Verification items for the finished model (mm, model axes). A direction names the side the tool comes from. Round coordinates to 2 decimals unless told otherwise and drop trailing zeros. Use CSV: the item, a comma, the result in double quotes.
```python
from build123d import *

# Parameters (mm, degrees)
SKETCH_1_R           = 155
EXTRUDE_1_DEPTH      = 5
SKETCH_3_R           = 6
CUT_EXTRUDE_3_DEPTH  = 10
SKETCH_7_R           = 21.5
CUT_EXTRUDE_7_DEPTH  = 10
SKETCH_8_R           = 1.5
CUT_EXTRUDE_8_DEPTH  = 7
SKETCH_12_R          = 1.5
CUT_EXTRUDE_12_DEPTH = 10
SKETCH_14_R          = 1.5
CUT_EXTRUDE_13_DEPTH = 220.260119493
SKETCH_15_R          = 1.5
SKETCH_15_W          = 120
SKETCH_15_H          = 25
CUT_EXTRUDE_14_DEPTH = 220.260119493
SKETCH_16_R          = 1.5
CUT_EXTRUDE_15_DEPTH = 220.260119493
SKETCH_17_R          = 3.25
CUT_EXTRUDE_16_DEPTH = 2
SKETCH_19_R          = 2
CUT_EXTRUDE_17_DEPTH = 220.260119493
SKETCH_20_R          = 1.5
CUT_EXTRUDE_18_DEPTH = 220.260119493
SKETCH_21_R          = 1.5
SKETCH_21_W          = 8
SKETCH_21_H          = 10
CUT_EXTRUDE_19_DEPTH = 220.260119493
SKETCH_23_R          = 2.5
SKETCH_23_W          = 6
SKETCH_23_H          = 7.5
CUT_EXTRUDE_20_DEPTH = 10


with BuildPart() as part:
    # Sketch 1 → Extrude 1 (new body)
    with BuildSketch(Plane.XY):
        Circle(SKETCH_1_R)
    extrude(amount=EXTRUDE_1_DEPTH)

    # Sketch 3 → Cut-Extrude 3 (cut)
    with BuildSketch(Plane.XY.offset(5)):
        with Locations((90, 90)):
            Circle(SKETCH_3_R)
        with Locations((-90, 90)):
            Circle(SKETCH_3_R)
    extrude(amount=-CUT_EXTRUDE_3_DEPTH, mode=Mode.SUBTRACT)

    # Sketch 7 → Cut-Extrude 7 (cut)
    with BuildSketch(Plane.XY.offset(5)):
        with Locations((0, 120)):
            Circle(SKETCH_7_R)
    extrude(amount=-CUT_EXTRUDE_7_DEPTH, mode=Mode.SUBTRACT)

    # Sketch 8 → Cut-Extrude 8 (cut)
    with BuildSketch(Plane.XY.offset(5)):
        with Locations((-20, 140)):
            Circle(SKETCH_8_R)
        with Locations((-20, 100)):
            Circle(SKETCH_8_R)
        with Locations((20, 100)):
            Circle(SKETCH_8_R)
        with Locations((20, 140)):
            Circle(SKETCH_8_R)
    extrude(amount=-CUT_EXTRUDE_8_DEPTH, mode=Mode.SUBTRACT)

    # Sketch 12 → Cut-Extrude 12 (cut)
    with BuildSketch(Plane.XY.offset(5)):
        with Locations((-90, 105)):
            Circle(SKETCH_12_R)
        with Locations((-77.009618943, 82.5)):
            Circle(SKETCH_12_R)
        with Locations((-102.990381057, 82.5)):
            Circle(SKETCH_12_R)
        with Locations((102.990381057, 82.5)):
            Circle(SKETCH_12_R)
        with Locations((77.009618943, 82.5)):
            Circle(SKETCH_12_R)
        with Locations((90, 105)):
            Circle(SKETCH_12_R)
    extrude(amount=-CUT_EXTRUDE_12_DEPTH, mode=Mode.SUBTRACT)

    # Sketch 14 → Cut-Extrude 13 (cut, through all)
    with BuildSketch(Plane.XY.offset(5)):
        with Locations((-80, -45)):
            Circle(SKETCH_14_R)
        with Locations(Location((-80, -51, 0), (0, 0, 180))):
            Circle(SKETCH_14_R)
        with Locations((80, -51)):
            Circle(SKETCH_14_R)
        with Locations(Location((80, -45, 0), (0, 0, 180))):
            Circle(SKETCH_14_R)
    extrude(amount=-CUT_EXTRUDE_13_DEPTH, mode=Mode.SUBTRACT)

    # Sketch 15 → Cut-Extrude 14 (cut, through all)
    with BuildSketch(Plane.XY.offset(5)):
        with Locations((-87, 51)):
            Circle(SKETCH_15_R)
        with Locations(Location((-77, 51, 0), (0, 0, 180))):
            Circle(SKETCH_15_R)
        with Locations((-77, 29)):
            Circle(SKETCH_15_R)
        with Locations(Location((-87, 29, 0), (0, 0, 180))):
            Circle(SKETCH_15_R)
        with Locations((0, 40)):
            Rectangle(SKETCH_15_W, SKETCH_15_H)
    extrude(amount=-CUT_EXTRUDE_14_DEPTH, mode=Mode.SUBTRACT)

    # Sketch 16 → Cut-Extrude 15 (cut, through all)
    with BuildSketch(Plane.XY.offset(5)):
        with Locations((0, 148)):
            Circle(SKETCH_16_R)
        with Locations((104.651803616, 104.651803616)):
            Circle(SKETCH_16_R)
        with Locations((148, 0)):
            Circle(SKETCH_16_R)
        with Locations((104.651803616, -104.651803616)):
            Circle(SKETCH_16_R)
        with Locations((0, -148)):
            Circle(SKETCH_16_R)
        with Locations((-104.651803616, -104.651803616)):
            Circle(SKETCH_16_R)
        with Locations((-148, 0)):
            Circle(SKETCH_16_R)
        with Locations((-104.651803616, 104.651803616)):
            Circle(SKETCH_16_R)
    extrude(amount=-CUT_EXTRUDE_15_DEPTH, mode=Mode.SUBTRACT)

    # Sketch 17 → Cut-Extrude 16 (cut)
    with BuildSketch(Plane(origin=(0, 0, 0), x_dir=(-1, 0, 0), z_dir=(0, 0, -1))):
        with Locations((-90, 105)):
            Circle(SKETCH_17_R)
        with Locations((-77.009618943, 82.5)):
            Circle(SKETCH_17_R)
        with Locations((-102.990381057, 82.5)):
            Circle(SKETCH_17_R)
        with Locations(Location((102.990381057, 82.5, 0), (0, 0, 180))):
            Circle(SKETCH_17_R)
        with Locations(Location((77.009618943, 82.5, 0), (0, 0, 180))):
            Circle(SKETCH_17_R)
        with Locations(Location((90, 105, 0), (0, 0, 180))):
            Circle(SKETCH_17_R)
    extrude(amount=-CUT_EXTRUDE_16_DEPTH, mode=Mode.SUBTRACT)

    # Sketch 19 → Cut-Extrude 17 (cut, through all)
    with BuildSketch(Plane(origin=(0, 0, 0), x_dir=(-1, 0, 0), z_dir=(0, 0, -1))):
        with Locations((-85.44, -26)):
            Circle(SKETCH_19_R)
        with Locations((-139, -36.5)):
            Circle(SKETCH_19_R)
        with Locations((-106, -94.5)):
            Circle(SKETCH_19_R)
        with Locations((106, -94.5)):
            Circle(SKETCH_19_R)
        with Locations((139, -36.5)):
            Circle(SKETCH_19_R)
        with Locations((85.44, -26)):
            Circle(SKETCH_19_R)
        with BuildLine():
            Line((92.5, -41.884919825), (92.5, -85.5))
            ThreePointArc((92.5, -85.5), (93.818019485, -88.681980515), (97, -90))
            Line((97, -90), (116, -90))
            ThreePointArc((116, -90), (119.181980515, -88.681980515), (120.5, -85.5))
            Line((120.5, -85.5), (120.5, -74.5))
            ThreePointArc((120.5, -74.5), (120.939339828, -73.439339828), (122, -73))
            Line((122, -73), (130, -73))
            ThreePointArc((130, -73), (133.181980515, -71.681980515), (134.5, -68.5))
            Line((134.5, -68.5), (134.5, -21.088475038))
            ThreePointArc((134.5, -21.088475038), (134.536795814, -20.45333724), (134.646690917, -19.826697774))
            ThreePointArc((134.646690917, -19.826697774), (137.219058182, -1.024043348), (136.174719632, 17.925))
            ThreePointArc((136.174719632, 17.925), (132.975444949, 23.703731672), (126.782202664, 26))
            Line((126.782202664, 26), (94, 26))
            ThreePointArc((94, 26), (90.818019485, 24.681980515), (89.5, 21.5))
            Line((89.5, 21.5), (89.5, -34.115080175))
            ThreePointArc((89.5, -34.115080175), (89.663282823, -35.316281294), (90.141281834, -36.430311075))
            Line((90.141281834, -36.430311075), (91.716211091, -39.05519317))
            ThreePointArc((91.716211091, -39.05519317), (92.300432105, -40.416785124), (92.5, -41.884919825))
        make_face()
        with BuildLine():
            Line((-91.716211091, -39.05519317), (-90.141281834, -36.430311075))
            ThreePointArc((-90.141281834, -36.430311075), (-89.663282823, -35.316281294), (-89.5, -34.115080175))
            Line((-89.5, -34.115080175), (-89.5, 21.5))
            ThreePointArc((-89.5, 21.5), (-90.818019485, 24.681980515), (-94, 26))
            Line((-94, 26), (-126.782202664, 26))
            ThreePointArc((-126.782202664, 26), (-132.975444949, 23.703731672), (-136.174719632, 17.925))
            ThreePointArc((-136.174719632, 17.925), (-137.219058182, -1.024043348), (-134.646690917, -19.826697774))
            ThreePointArc((-134.646690917, -19.826697774), (-134.536795814, -20.45333724), (-134.5, -21.088475038))
            Line((-134.5, -21.088475038), (-134.5, -68.5))
            ThreePointArc((-134.5, -68.5), (-133.181980515, -71.681980515), (-130, -73))
            Line((-130, -73), (-122, -73))
            ThreePointArc((-122, -73), (-120.939339828, -73.439339828), (-120.5, -74.5))
            Line((-120.5, -74.5), (-120.5, -85.5))
            ThreePointArc((-120.5, -85.5), (-119.181980515, -88.681980515), (-116, -90))
            Line((-116, -90), (-97, -90))
            ThreePointArc((-97, -90), (-93.818019485, -88.681980515), (-92.5, -85.5))
            Line((-92.5, -85.5), (-92.5, -41.884919825))
            ThreePointArc((-92.5, -41.884919825), (-92.300432105, -40.416785124), (-91.716211091, -39.05519317))
        make_face()
    extrude(amount=-CUT_EXTRUDE_17_DEPTH, mode=Mode.SUBTRACT)

    # Sketch 20 → Cut-Extrude 18 (cut, through all)
    with BuildSketch(Plane(origin=(0, 0, 0), x_dir=(-1, 0, 0), z_dir=(0, 0, -1))):
        with Locations((-79, -15)):
            Circle(SKETCH_20_R)
        with Locations((79, -15)):
            Circle(SKETCH_20_R)
    extrude(amount=-CUT_EXTRUDE_18_DEPTH, mode=Mode.SUBTRACT)

    # Sketch 21 → Cut-Extrude 19 (cut, through all)
    with BuildSketch(Plane(origin=(0, 0, 0), x_dir=(-1, 0, 0), z_dir=(0, 0, -1))):
        with Locations((-52, 58.5)):
            Circle(SKETCH_21_R)
        with Locations((0, 58.5)):
            Circle(SKETCH_21_R)
        with Locations((52, 58.5)):
            Circle(SKETCH_21_R)
        with Locations((-66, 57.5)):
            Rectangle(SKETCH_21_W, SKETCH_21_H)
        with Locations((-66, 22.5)):
            Rectangle(SKETCH_21_W, SKETCH_21_H)
        with Locations((66, 22.5)):
            Rectangle(SKETCH_21_W, SKETCH_21_H)
        with Locations((66, 57.5)):
            Rectangle(SKETCH_21_W, SKETCH_21_H)
    extrude(amount=-CUT_EXTRUDE_19_DEPTH, mode=Mode.SUBTRACT)

    # Sketch 23 → Cut-Extrude 20 (cut)
    with BuildSketch(Plane.XY.offset(5)):
        with Locations((5, 150)):
            Circle(SKETCH_23_R)
        Polygon((71.094872981, 133.139932161), (68.169872981, 128.073683549), (76.830127019, 123.073683549), (79.755127019, 128.139932161), align=None)
        Polygon((128.139932161, 79.755127019), (123.073683549, 76.830127019), (128.073683549, 68.169872981), (133.139932161, 71.094872981), align=None)
        with Locations((-6, 150)):
            Rectangle(SKETCH_23_W, SKETCH_23_H)
        Polygon((79.755127019, -128.139932161), (76.830127019, -123.073683549), (68.169872981, -128.073683549), (71.094872981, -133.139932161), align=None)
        Polygon((-71.094872981, -133.139932161), (-68.169872981, -128.073683549), (-76.830127019, -123.073683549), (-79.755127019, -128.139932161), align=None)
        Polygon((-133.139932161, 71.094872981), (-128.073683549, 68.169872981), (-123.073683549, 76.830127019), (-128.139932161, 79.755127019), align=None)
        Polygon((-79.755127019, 128.139932161), (-76.830127019, 123.073683549), (-68.169872981, 128.073683549), (-71.094872981, 133.139932161), align=None)
    extrude(amount=-CUT_EXTRUDE_20_DEPTH, mode=Mode.SUBTRACT)


solid = part.part
```
Q1. Access from +Z, -Z, +X, -X, +Y, -Y to the whole of each face (thin tool, end or side, straight path). Record for faces 1 (the flat face through (-2, 2, 5)), 2 (the cylindrical face through (132.904, 23.765, 2.465)).
Filled in:
face 1,"+Z, +X, -X, +Y, -Y"
face 2,"+Z, -Z"
Q2. Section check A-A (z = 3.4). State how many separate pieces and enclosed holes the cut face has, plus the area to 3 significant figures.
Filled in:
separate pieces,"1"
enclosed holes,"55"
area,"60,000 mm²"
Q3. Material ranges on L1, parallel to X at y = -3.5, z = 2.45; L2, parallel to X at y = -77, z = 4.8; L3, parallel to X at y = 82.5, z = 3.15, recorded low to high.
Filled in:
L1,"-154.96 to -137.09, -89.5 to 89.5, 137.09 to 154.96"
L2,"-134.52 to -120.5, -92.5 to 92.5, 120.5 to 134.52"
L3,"-131.22 to -104.49, -101.49 to -78.51, -75.51 to 75.51, 78.51 to 101.49, 104.49 to 131.22"
Q4. Mould release check, pull along Y, two halves, no side actions. Record for faces 3 (the cylindrical face through (-33.601, -151.314, 2.465)), 4 (the cylindrical face through (-94.42, 94.06, 2.54)), 5 (the flat face through (-2, 2, 0)): released by +Y, released by -Y, zero draft, split by the parting line, or undercut.
Filled in:
face 3,"split by the parting line"
face 4,"undercut"
face 5,"zero draft"
Q5. Go/stop test with flat-tipped pins: P1, Ø2.5, axis at y = 57.5, z = 3, coming from the -X side; P2, Ø2, axis at y = 75.5, z = 3.5, coming from the +X side; P3, Ø2, axis at y = 122.5, z = 4, coming from the -X side. Record where each tip stops, or that it passes through.
Filled in:
P1,"x = -144.43"
P2,"x = 135.92"
P3,"x = -96.24"
